The listing builds one solid part. Answer for the finished solid, in the listing's coordinates (mm). A direction names the side the tool comes from. Round coordinates to 2 decimals unless told otherwise and drop trailing zeros. Order: outer loops, then holes, each group sorted by start corner. A loop starts at its lowest first (then second) coordinate and runs counter-clockwise, first axis right, second up. Notation, with made-up numbers: (-8, -28) - (11, -28) arc R35 ccw to (11, 5) - close; hole circle Ø3 at (-4, -20). An arc over 180 degrees is marked (long way). One line per item, written item: value. Start each with the question number.
1. Flat-ended cylindrical pins translate along their axes: P1, Ø15, axis at x = 145, z = -90.5, coming from the +Y side; P2, Ø11, axis at x = -7.5, y = -3.5, coming from the +Z side; P3, Ø3, axis at y = 3, z = -11, coming from the -X side. Find the tip coordinate at first contact, or state that the pin passes through.
2. For a pull along Z with two mould halves and no side action, classify faces 4 (the flat face through (14, 4, -69)), 5 (the flat face through (85, 3, -140)), 6 (the flat face through (122, 6, -55)), 7 (the flat face through (-6, 0, -30)) as released by +Z, released by -Z, zero draft, split by the parting line, or undercut.
3. A tool of negligible diameter and unlimited length cuts with its end or side. For faces 1 (the flat face through (-6, 0, -110)), 2 (the cylindrical face through (122.25, 9.77, -112.12)), 3 (the flat face through (123, 7, -85)), from which of +Z, -Z, +X, -X, +Y, -Y can it reach the whole face along a straight path? Write none if from no direction.
4. Section D-D, the plane z = -11 is taken. Give the vertices of the cut face in (x, y) (1 decimal).
5. Section A-A, the plane z = -66.5 is taken. Give the vertices of the cut face in (x, y), then the cut area to 3 significant figures.
6. Section B-B, the plane x = 92 is taken. Give the vertices of the cut face in (y, z), then the cut area to 3 significant figures.
7. Straight lines are drawn through the part: line 1 (Y direction, x = -7.5, z = -79.5); line 2 (Z direction, x = 87, y = 3.5); line 3 (Y direction, x = 99.5, z = -18). For each, find the intervals that lie inside material, in ascending order.
8. Section C-C, the plane y = -3.5 is taken. Give the vertices of the cut face in (x, z).
from build123d import *

# Parameters (mm, degrees)
SKETCH_1_R               = 3.5
EXTRUDE_1_DEPTH          = 140
SKETCH_2_W               = 30
SKETCH_2_H               = 27.344925094
CUT_EXTRUDE_1_DEPTH      = 214.393529953
CUT_EXTRUDE_3_DEPTH      = 214.005050566
CUT_EXTRUDE_3_DEPTH_BACK = 214.005050566


with BuildPart() as part:
    # 草图1 → 凸台-拉伸1 (new body)
    with BuildSketch(Plane.XY):
        with BuildLine():
            Line((154.968701019, 4), (124.968701019, 4))
            ThreePointArc((124.968701019, 4), (127.137930645, 14.150809034), (120.852941176, 22.411764706))
            ThreePointArc((120.852941176, 22.411764706), (117.470588235, 21.382352941), (118.5, 18))
            ThreePointArc((118.5, 18), (122.215434845, 9.633641289), (115, 4))
            Line((115, 4), (0, 4))
            Line((0, 4), (-7.5, 4))
            ThreePointArc((-7.5, 4), (-11.372983346, -9.922616289), (-0.866750419, 0))
            Line((-0.866750419, 0), (0, 0))
            Line((0, 0), (115, 0))
            Line((115, 0), (159.440401192, 0))
            ThreePointArc((159.440401192, 0), (157.968538616, 2.854080771), (154.968701019, 4))
        make_face()
        with Locations((-7.5, -3.5)):
            Circle(SKETCH_1_R, mode=Mode.SUBTRACT)
    extrude(amount=-EXTRUDE_1_DEPTH)

    # 草图2 → 切除-拉伸1 (cut, through all)
    with BuildSketch(Plane(origin=(0, 0, 0), x_dir=(0, 0, -1), z_dir=(1, 0, 0))):
        with Locations((15, -2.172462547)):
            Rectangle(SKETCH_2_W, SKETCH_2_H)
        with Locations((125, -2.172462547)):
            Rectangle(SKETCH_2_W, SKETCH_2_H)
    extrude(amount=-CUT_EXTRUDE_1_DEPTH, mode=Mode.SUBTRACT)

    # 草图3 → 切除-拉伸3 (cut, two sides: drawn at the far end of the back side and taken through both)
    with BuildSketch(Plane(origin=(0, 4, 0), x_dir=(1, 0, 0), z_dir=(0, 1, 0)).offset(-CUT_EXTRUDE_3_DEPTH_BACK)):
        with BuildLine():
            Line((15, 106.057196128), (15, 33.942803872))
            ThreePointArc((15, 33.942803872), (19.815985752, 22.315985752), (31.442803872, 17.5))
            Line((31.442803872, 17.5), (95.059923468, 17.5))
            ThreePointArc((95.059923468, 17.5), (98.553085083, 18.946914917), (100, 22.440076532))
            Line((100, 22.440076532), (100, 50))
            ThreePointArc((100, 50), (101.464466094, 53.535533906), (105, 55))
            Line((105, 55), (115, 55))
            Line((115, 55), (137.57175482, 55))
            ThreePointArc((137.57175482, 55), (142.824317359, 57.175682641), (145, 62.42824518))
            Line((145, 62.42824518), (145, 77.57175482))
            ThreePointArc((145, 77.57175482), (142.824317359, 82.824317359), (137.57175482, 85))
            Line((137.57175482, 85), (115, 85))
            Line((115, 85), (105, 85))
            ThreePointArc((105, 85), (101.464466094, 86.464466094), (100, 90))
            Line((100, 90), (100, 117.559923468))
            ThreePointArc((100, 117.559923468), (98.553085083, 121.053085083), (95.059923468, 122.5))
            Line((95.059923468, 122.5), (31.442803872, 122.5))
            ThreePointArc((31.442803872, 122.5), (19.815985752, 117.684014248), (15, 106.057196128))
        make_face()
    extrude(amount=CUT_EXTRUDE_3_DEPTH + CUT_EXTRUDE_3_DEPTH_BACK, mode=Mode.SUBTRACT)


solid = part.part
Answer list:
1. P1: stops at y = 4
1. P2: stops at z = -30
1. P3: stops at x = 0
2. face 4: zero draft
2. face 5: released by -Z
2. face 6: undercut
2. face 7: released by +Z
3. face 1: -Z, -X, +Y, -Y
3. face 2: +Z, -Z, -X
3. face 3: +Y, -Y
4. outline: (0, 0) - (159.4, 0) arc R4.5 ccw to (155, 4) - (125, 4) arc R12.4 ccw to (120.9, 22.4) arc R2.5 ccw to (118.5, 18) arc R7.4 cw to (115, 4) - (0, 4) - close
5. outline: (-7.5, 4) arc R7.5 ccw (long way) to (-0.87, 0) - (15, 0) - (15, 4) - close; (145, 0) - (159.44, 0) arc R4.5 ccw to (154.97, 4) - (145, 4) - close; hole circle Ø7 at (-7.5, -3.5)
5. area: 263 mm²
6. outline: (0, -140) - (4, -140) - (4, -122.5) - (0, -122.5) - close; (0, -17.5) - (4, -17.5) - (4, 0) - (0, 0) - close
6. area: 140 mm²
7. line 1: y = -11 to -7, 0 to 4
7. line 2: z = -140 to -122.5, -17.5 to 0
7. line 3: y = 0 to 4
8. outline: (-15, -110) - (-11, -110) - (-11, -30) - (-15, -30) - close; (-4, -110) - (0, -110) - (0, -30) - (-4, -30) - close
